Could you check a few things on this model? Use its own coordinates, in mm. A direction names the side the tool comes from. Give positions to 0.01 mm unless a question says otherwise; leave off trailing zeros. Loops run counter-clockwise (first coordinate to the right, second up) from the corner with the lowest first, then second, coordinate; pieces in that order, holes last. Notation, with made-up numbers: (78.25, -36) - (135.25, -36) arc R19 cw to (135.25, -8) - close; hole circle Ø6 at (45, -4.75). An arc over 180 degrees is marked (long way). One line per item, written item: value. Start each with the question number.
Q1. If I drill on line 1 (X direction, y = -3.6, z = 0); line 2 (X direction, y = 0.5, z = -2.25); line 3 (Y direction, x = -6.5, z = 2) (3 decimals), over which ranges is the centre line in solid material (lowest first)? Write a range as from..to.
Q2. For faces 1 (the face through (0, 0, 3)), 2 (the face through (-23.036, -3, -3)), 3 (the face through (-38.276, 2, -3)), which set-ups out of +Z, -Z, +X, -X, +Y, -Y let a thin tool reach every point of the face, with its end or its side?
Q3. I want a section at D-D (y = -2). Please give me the cut outline in (x, z).
Q4. I want a section at C-C (x = 13.5). Please give me the cut outline in (y, z) (3 decimals), then the cut area to 3 significant figures.
Q5. I want a section at B-B (y = 0). Please give me the cut outline in (x, z) (3 decimals).
Q6. If we mould it in two halves opening along X, with no side actions, what happens to faces 4 (the face through (-36.74, -3.39, -0.33)), 5 (the face through (11, -2, -4)), 6 (the face through (-12, 4.365, 0))? For each: released by +X, released by -X, zero draft, split by the parting line, or undercut.
Q7. I'm going to push flat-ended pins straight in: P1, Ø1.5, axis at x = -12.5, z = -0.5, coming from the +Y side (3 decimals); P2, Ø1, axis at x = -19, y = 3.5, coming from the +Z side; P3, Ø0.5, axis at y = 5, z = -0.5, coming from the -X side; P4, Ø5, axis at y = 0, z = 1.5, coming from the -X side. Where does each tip first touch, or does it pass through?
Q8. I want a section at A-A (z = 0). Please give me the cut outline in (x, y) (3 decimals).
```python
from build123d import *

# Parameters (mm, degrees)
SKETCH8_R          = 1.5
CUT_EXTRUDE2_DEPTH = 10
SKETCH9_R          = 3.17
CUT_EXTRUDE3_DEPTH = 7
SKETCH10_R         = 3
CUT_EXTRUDE4_DEPTH = 32.5
SKETCH12_W         = 24.803289192
SKETCH12_H         = 5.136244689
CUT_EXTRUDE5_DEPTH = 12.7


with BuildPart() as part:
    # Sketch6 → Revolve1 (revolve)
    with BuildSketch(Plane.XY, mode=Mode.PRIVATE) as revolve1_sk:
        Polygon((-38.276, 0), (-38.276, 4.005), (-23.036, 4.005), (-23.036, 5), (11, 5), (11, 4.005), (16, 4.005), (16, 0), align=None)
    revolve(revolve1_sk.sketch.rotate(Axis((-1000, 0, 0), (1, 0, 0)), 90), axis=Axis((-1000, 0, 0), (1, 0, 0)))

    # Sketch8 → Cut-Extrude2 (cut)
    with BuildSketch(Plane(origin=(0, 0, 0), x_dir=(1, 0, 0), z_dir=(0, 1, 0))):
        with Locations(Location((-35.276, 0, 0), (0, 0, 270))):
            Circle(SKETCH8_R)
    extrude(amount=-CUT_EXTRUDE2_DEPTH, mode=Mode.SUBTRACT)

    # Sketch9 → Cut-Extrude3 (cut)
    with BuildSketch(Plane.ZY.offset(38.276)):
        Circle(SKETCH9_R)
    extrude(amount=-CUT_EXTRUDE3_DEPTH, mode=Mode.SUBTRACT)

    # Sketch10 → Cut-Extrude4 (cut)
    with BuildSketch(Plane(origin=(16, 0, 0), x_dir=(0, 0, -1), z_dir=(1, 0, 0))):
        Circle(SKETCH10_R)
    extrude(amount=-CUT_EXTRUDE4_DEPTH, mode=Mode.SUBTRACT)

    # Sketch12 → Cut-Extrude5 (cut, symmetric)
    with BuildSketch(Plane.XY):
        with Locations((-13.109401935, 6.933122345)):
            Rectangle(SKETCH12_W, SKETCH12_H)
    extrude(amount=CUT_EXTRUDE5_DEPTH, both=True, mode=Mode.SUBTRACT)


solid = part.part
```
Worked answers:
1. line 1: x = -38.28..-36.78, -33.78..16
1. line 2: x = -31.28..-16.5
1. line 3: y = -4.583..-2.236, 2.236..4.365
2. face 1: +X
2. face 2: -X
2. face 3: +Z, -Z, -X, +Y, -Y
3. outline: (-38.28, -3.47) - (-23.04, -3.47) - (-23.04, -4.58) - (11, -4.58) - (11, -3.47) - (16, -3.47) - (16, -2.24) - (-16.5, -2.24) - (-16.5, 2.24) - (16, 2.24) - (16, 3.47) - (11, 3.47) - (11, 4.58) - (-23.04, 4.58) - (-23.04, 3.47) - (-38.28, 3.47) - (-38.28, 2.46) - (-31.28, 2.46) - (-31.28, -2.46) - (-38.28, -2.46) - close
4. outline: circle Ø8.01 at (0, 0); hole circle Ø6 at (0, 0)
4. area: 22.1 mm²
5. outline: (-38.276, -4.005) - (-23.036, -4.005) - (-23.036, -5) - (11, -5) - (11, -4.005) - (16, -4.005) - (16, -3) - (-16.5, -3) - (-16.5, 3) - (16, 3) - (16, 4.005) - (11, 4.005) - (11, 5) - (-23.036, 5) - (-23.036, 4.005) - (-38.276, 4.005) - (-38.276, 3.17) - (-31.276, 3.17) - (-31.276, -3.17) - (-38.276, -3.17) - close
6. face 4: undercut
6. face 5: released by +X
6. face 6: zero draft
7. P1: stops at y = 4.365
7. P2: stops at z = 4
7. P3: stops at x = -0.71
7. P4: stops at x = -38.28
8. outline: (-38.276, -4.005) - (-36.776, -4.005) - (-36.776, -3.17) - (-38.276, -3.17) - close; (-38.276, 3.17) - (-31.276, 3.17) - (-31.276, -3.17) - (-33.776, -3.17) - (-33.776, -4.005) - (-23.036, -4.005) - (-23.036, -5) - (11, -5) - (11, -4.005) - (16, -4.005) - (16, -3) - (-16.5, -3) - (-16.5, 3) - (16, 3) - (16, 4.005) - (11, 4.005) - (11, 5) - (-0.708, 5) - (-0.708, 4.365) - (-23.036, 4.365) - (-23.036, 4.005) - (-38.276, 4.005) - close
